Geometry check sheet. Reference: the model listing, model coordinates, mm. A direction names the side the tool comes from. Coordinates: 2 decimals unless noted, no trailing zeros. Order: outer loops, then holes, each group sorted by start corner. A loop starts at its lowest first (then second) coordinate and runs counter-clockwise, first axis right, second up. Notation, with made-up numbers: (-16.75, 84) -> (24.25, 84) arc R12 cw to (24.25, 97) -> close; hole circle Ø5 at (18, 43). An arc over 180 degrees is marked (long way). Answer in a Markdown table with one row per item. Add a question column.
```python
from build123d import *

# Parameters (mm, degrees)
F1_DEPTH = 76.2
F3_DEPTH = 107.7030838857
F5_W     = 15.6415318966
F5_H     = 54.425964132
F6_DEPTH = 25.4
F8_DEPTH = 149.6723981032


# Not quite as in the source:
# - a feature of the source that left no trace in its solid (it failed there, or was rolled back) is left out


with BuildPart() as f1:
    # F0 (on Front) → F1 (new body)
    with BuildSketch(Plane.XZ):
        Polygon((55.1925264299, 74.4524151087), (31.4290784299, 74.4524151087), (31.4290784299, -56.2465488911), (-52.5095574558, -56.2465488911), (-52.5095574558, -75.2189829946), (55.1925264299, -75.2189829946), align=None)
    extrude(amount=F1_DEPTH)

    # F2 (on face) → F3 (cut, through all)
    with BuildSketch(Plane.YZ.offset(55.1925264299)):
        with BuildLine():
            Line((-47.1170713552, 8.9112932328), (-29.1559303752, 8.9112932328))
            ThreePointArc((-29.1559303752, 8.9112932328), (-38.1365008652, 17.8918637228), (-47.1170713552, 8.9112932328))
        make_face()
        with BuildLine():
            ThreePointArc((-47.1170713552, 8.9112932328), (-38.1365008652, -0.0692772572), (-29.1559303752, 8.9112932328))
            Line((-29.1559303752, 8.9112932328), (-47.1170713552, 8.9112932328))
        make_face()
        with BuildLine():
            ThreePointArc((-47.1170713552, 8.9112932328), (-38.1365008652, 17.8918637228), (-29.1559303752, 8.9112932328))
            Line((-29.1559303752, 8.9112932328), (-28.9377495646, 8.9112932328))
            Line((-28.9377495646, 8.9112932328), (-28.9377495646, 74.4524151087))
            Line((-28.9377495646, 74.4524151087), (-47.1170713552, 74.4524151087))
            Line((-47.1170713552, 74.4524151087), (-47.1170713552, 8.9112932328))
        make_face()
    extrude(amount=-F3_DEPTH, mode=Mode.SUBTRACT)

    # F5 (on face) → F6 (cut)
    with BuildSketch(Plane.YZ.offset(55.1925264299)):
        with Locations((-68.3792340517, -48.0060009286)):
            Rectangle(F5_W, F5_H)
    extrude(amount=-F6_DEPTH, mode=Mode.SUBTRACT)

    # F7 (on face) → F8 (cut, through all)
    with BuildSketch(Plane(origin=(0, 0, -75.2189829946), x_dir=(1, 0, 0), z_dir=(0, 0, -1))):
        with BuildLine():
            ThreePointArc((-17.3657385867, 0), (-52.4302228968, 39.5091264656), (-14.1626540173, 75.9245394945))
            Line((-14.1626540173, 75.9245394945), (-14.1626540173, 76.2))
            Line((-14.1626540173, 76.2), (-52.5095574558, 76.2))
            Line((-52.5095574558, 76.2), (-52.5095574558, 0))
            Line((-52.5095574558, 0), (-17.3657385867, 0))
        make_face()
    extrude(amount=-F8_DEPTH, mode=Mode.SUBTRACT)


solid = f1.part
```
(1) Cross-section at D-D (z = -30). Enter the section's corners in (x, y).
(2) Go/stop test with flat-tipped pins: P1, Ø7.5, axis at x = 37, z = -46, coming from the -Y side; P2, Ø17, axis at y = -70, z = -64, coming from the +X side; P3, Ø1.5, axis at y = -59, z = 46.5, coming from the -X side. Record where each tip stops, or that it passes through.
(3) Access from +Z, -Z, +X, -X, +Y, -Y to the whole of each face (thin tool, end or side, straight path). Record for faces 5 (the face through (43, -60.558, -48)), 6 (the face through (29.793, -68, -66)), 7 (the face through (43, -28.938, 41)).
(4) Mould release check, pull along Y, two halves, no side actions. Record for faces 1 (the face through (43, -47.117, 42)), 2 (the face through (55.193, -38, -1)), 3 (the face through (43.477, -38.334, -0.067)), 4 (the face through (-52.456, -38.692, -65.866)): +Y half, -Y half, draft (parallel to the pull), parting line (faces both ways), or undercut.
(5) Scan lines: line 1 along Y through (x, z) = (49.5, 28); line 2 along X through (y, z) = (-16.5, 41.5); line 3 along Z through (x, y) = (3, -19). Record each from-to range of solid material in increasing order.
(6) Cross-section at A-A (z = 61.5). Enter the section's corners in (x, y), plus the area to 3 significant figures.
(7) Cross-section at B-B (x = -9.5). Enter the section's corners in (y, z).
(8) Cross-section at C-C (y = -39.5). Enter the section's corners in (x, z).
Checks:
| question | item | result |
|---|---|---|
| 1 | outline | (31.43, -60.56) -> (55.19, -60.56) -> (55.19, 0) -> (31.43, 0) -> close |
| 2 | P1 | y = -60.56 |
| 2 | P2 | x = 29.79 |
| 2 | P3 | x = 31.43 |
| 3 | face 5 | -Z, +X, -Y |
| 3 | face 6 | +Z, -Z, +X, -Y |
| 3 | face 7 | +Z, +X, -X |
| 4 | face 1 | undercut |
| 4 | face 2 | draft |
| 4 | face 3 | undercut |
| 4 | face 4 | parting line |
| 5 | line 1 | -76.2 to -47.12, -28.94 to 0 |
| 5 | line 2 | 31.43 to 55.19 |
| 5 | line 3 | -75.22 to -56.25 |
| 6 | outline | (31.43, -76.2) -> (55.19, -76.2) -> (55.19, -47.12) -> (31.43, -47.12) -> close; (31.43, -28.94) -> (55.19, -28.94) -> (55.19, 0) -> (31.43, 0) -> close |
| 6 | area | 1,380 mm² |
| 7 | outline | (-76.2, -75.22) -> (0, -75.22) -> (0, -56.25) -> (-76.2, -56.25) -> close |
| 8 | outline | (-52.43, -75.22) -> (55.19, -75.22) -> (55.19, 0.03) -> (31.43, 0.03) -> (31.43, -56.25) -> (-52.43, -56.25) -> close |
